Check sheet for the modelled part. Datum: model origin and axes. Units: mm. A direction names the side the tool comes from. Give positions to 0.01 mm unless a question says otherwise; leave off trailing zeros. Loops run counter-clockwise (first coordinate to the right, second up) from the corner with the lowest first, then second, coordinate; pieces in that order, holes last. Notation, with made-up numbers: (36.25, 1) - (75.25, 1) arc R37 ccw to (75.25, 37) - close; hole circle Ø1 at (17, -36). An arc over 180 degrees is marked (long way). Use one line per item in the form item = value.
from build123d import *

# Parameters (mm, degrees)
SKETCH_15_W         = 10
SKETCH_15_H         = 20
SKETCH_15_W_2       = 6
SKETCH_15_H_2       = 16
F_20X10X2_2_DEPTH   = 270
SKETCH_12_R         = 1.6
CUT_EXTRUDE_1_DEPTH = 271.370116692
SKETCH_16_R         = 6
CUT_EXTRUDE_2_DEPTH = 271.370116692
SKETCH_17_R         = 4
CUT_EXTRUDE_3_DEPTH = 18
SKETCH_18_R         = 1.6
CUT_EXTRUDE_4_DEPTH = 10


with BuildPart() as part:
    # 草图15 → 铝方管 20X10X2(2) (new body)
    with BuildSketch(Plane(origin=(0, 0, 0), x_dir=(0, 0, -1), z_dir=(1, 0, 0))):
        Rectangle(SKETCH_15_W, SKETCH_15_H)
        Rectangle(SKETCH_15_W_2, SKETCH_15_H_2, mode=Mode.SUBTRACT)
    extrude(amount=F_20X10X2_2_DEPTH)

    # 草图12 → 切除-拉伸1 (cut, through all)
    with BuildSketch(Plane.XY.offset(5)):
        with Locations((10, 0)):
            Circle(SKETCH_12_R)
        with Locations(Location((260, 0, 0), (0, 0, 180))):
            Circle(SKETCH_12_R)
    extrude(amount=-CUT_EXTRUDE_1_DEPTH, mode=Mode.SUBTRACT)

    # 草图16 → 切除-拉伸2 (cut, through all)
    with BuildSketch(Plane.XY.offset(5)):
        with Locations((60, 0)):
            Circle(SKETCH_16_R)
        with Locations(Location((210, 0, 0), (0, 0, 180))):
            Circle(SKETCH_16_R)
    extrude(amount=-CUT_EXTRUDE_2_DEPTH, mode=Mode.SUBTRACT)

    # 草图17 → 切除-拉伸3 (cut)
    with BuildSketch(Plane.XY.offset(5)):
        with Locations((135, 0)):
            Circle(SKETCH_17_R)
    extrude(amount=-CUT_EXTRUDE_3_DEPTH, mode=Mode.SUBTRACT)

    # 草图18 → 切除-拉伸4 (cut)
    with BuildSketch(Plane.XY.offset(5)):
        with Locations((120, 0)):
            Circle(SKETCH_18_R)
        with Locations((150, 0)):
            Circle(SKETCH_18_R)
    extrude(amount=-CUT_EXTRUDE_4_DEPTH, mode=Mode.SUBTRACT)


solid = part.part
Item 1: Mould release check, pull along Y, two halves, no side actions. Record for faces 1 (the face through (133, -10, 0)), 2 (the face through (138.815, 1.201, -3.986)), 3 (the face through (133, 4, -5)), 4 (the face through (133, -4, -3)): released by +Y, released by -Y, zero draft, split by the parting line, or undercut.
Answer block:
face_1 = released by -Y
face_2 = undercut
face_3 = zero draft
face_4 = undercut
Item 2: Gauge pin test, flat end, axial feed: P1, Ø5, axis at x = 150, y = 0, coming from the +Z side. Record the tip position at first contact, or that the pin passes through.
Answer block:
P1 = 5
Item 3: Access from +Z, -Z, +X, -X, +Y, -Y to the whole of each face (thin tool, end or side, straight path). Record for faces 5 (the face through (133, -4, 3)), 6 (the face through (138.815, 1.201, 4.014)).
Answer block:
face_5 = +X, -X
face_6 = +Z, -Z
Item 4: Thickness scan on L1, parallel to Z at x = 164, y = -0.25; L2, parallel to Y at x = 135, z = -4.25; L3, parallel to X at y = 2.75, z = -4.5. Record the ranges inside material, lowest first.
Answer block:
L1 = -5 to -3, 3 to 5
L2 = -10 to -4, 4 to 10
L3 = 0 to 54.67, 65.33 to 132.1, 137.9 to 204.67, 215.33 to 270
Item 5: Section check A-A on x = 60. Record the boundary of the cut face in (y, z).
Answer block:
outline = (-10, -5) - (-6, -5) - (-6, -3) - (-8, -3) - (-8, 3) - (-6, 3) - (-6, 5) - (-10, 5) - close; (6, -5) - (10, -5) - (10, 5) - (6, 5) - (6, 3) - (8, 3) - (8, -3) - (6, -3) - close
Item 6: Section check B-B on z = -0.5. Record the boundary of the cut face in (x, y).
Answer block:
outline = (0, -10) - (270, -10) - (270, -8) - (0, -8) - close; (0, 8) - (270, 8) - (270, 10) - (0, 10) - close
Item 7: Section check C-C on x = 250. Record the boundary of the cut face in (y, z), then the cut area to 3 significant figures.
Answer block:
outline = (-10, -5) - (10, -5) - (10, 5) - (-10, 5) - close; hole (-8, -3) - (8, -3) - (8, 3) - (-8, 3) - close
area = 104 mm2
